Geometry check sheet. Reference: the model listing, model coordinates, mm. Coordinates: 2 decimals unless noted, no trailing zeros. Loops run counter-clockwise (first coordinate to the right, second up) from the corner with the lowest first, then second, coordinate; pieces in that order, holes last.
from build123d import *

# Parameters (mm, degrees)
SKETCH1_R           = 9.3
BOSS_EXTRUDE1_DEPTH = 65.2
FILLET1_R           = 0.5


with BuildPart() as part:
    # Sketch1 → Boss-Extrude1 (new body)
    with BuildSketch(Plane.XY):
        Circle(SKETCH1_R)
    extrude(amount=-BOSS_EXTRUDE1_DEPTH)

    # Sketch3 → Cut-Revolve1 (revolve, cut)
    with BuildSketch(Plane(origin=(0, 0, 0), x_dir=(0, 0, -1), z_dir=(1, 0, 0))):
        Polygon((0, 5.89), (0, 3.775), (3, 5.89), align=None)
    revolve(axis=Axis((0, 0, 55), (0, 0, -1)), mode=Mode.SUBTRACT)

    # Fillet1
    fillet1_edges = [part.edges().sort_by_distance(p)[0] for p in [
        (-9.3, 0, 0),
        (-9.3, 0, -65.2),
    ]]
    fillet(fillet1_edges, radius=FILLET1_R)


solid = part.part
(1) Sectioned sample at A-A on z = -43. Record the cut outline in (x, y), and give its area (3 significant figures).
Findings:
outline: circle Ø18.6 at (0, 0)
area: 272 mm2
(2) Draft check along X on faces 1 (the cylindrical face through (5, 7.84, -32.15)), 2 (the flat face through (0, 0, -65.2)), 3 (the conical face through (-3.814, -0.847, -0.188)), 4 (the cylindrical face through (5.84, -0.77, -1.48)). Enter one of: +X half, -X half, draft (parallel to the pull), parting line (faces both ways), or undercut.
Findings:
face 1: parting line
face 2: draft
face 3: undercut
face 4: undercut
(3) Gauge pin test, flat ends, axial feed: pin 1 Ø1 at (x, z) = (5, -55.5) entering from -Y; pin 2 Ø8 at (x, z) = (-5.5, -11.5) entering from +Y; pin 3 Ø1.5 at (x, z) = (-4, -49.5) entering from +Y; pin 4 Ø8 at (x, z) = (-3, -42) entering from -Y. Record the tip position at first contact, or that the pin passes through.
Findings:
pin 1: stops at y = -8.14
pin 2: stops at y = 9.18
pin 3: stops at y = 8.71
pin 4: stops at y = -9.3
(4) Scan lines: L1, parallel to Z at x = 3.75, y = -0.5; L2, parallel to X at y = -8, z = -7; L3, parallel to Y at x = 5, z = -41.5. Record each from-to range of solid material in increasing order.
Findings:
L1: z = -65.2 to -0.01
L2: x = -4.74 to 4.74
L3: y = -7.84 to 7.84
